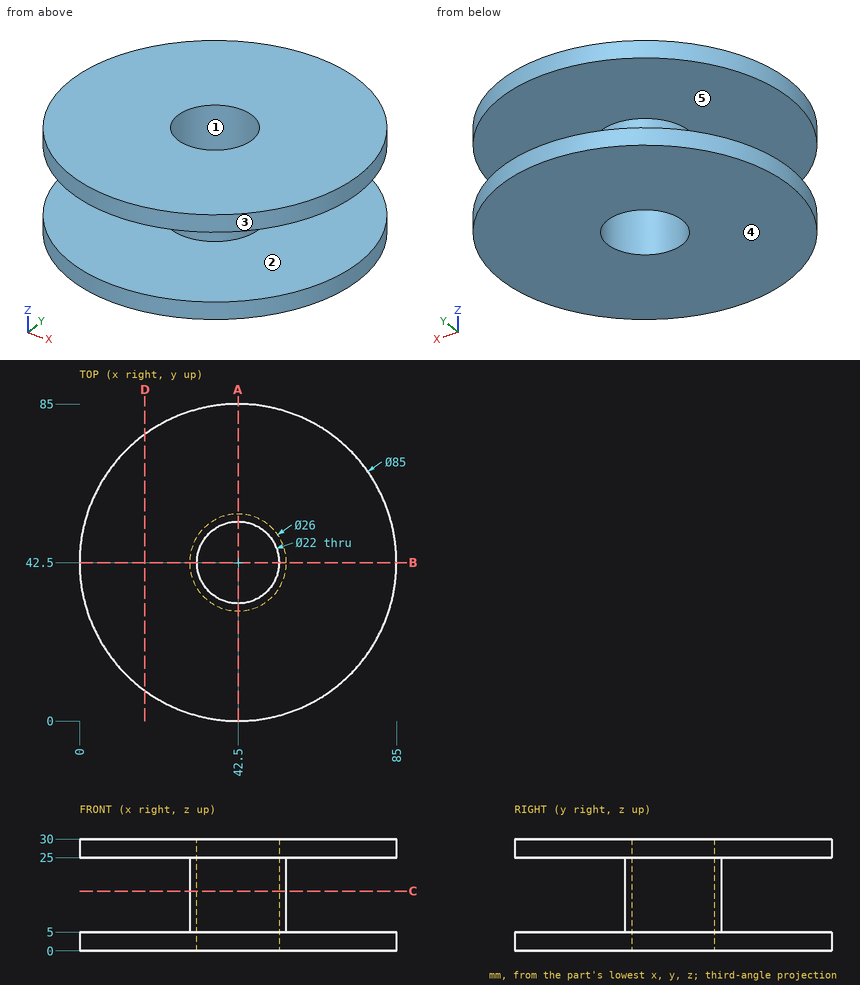
Here's the drawing with two shaded views (mm, measured from the low corner). I have some questions. A direction names the side the tool comes from. Coordinates: 2 decimals unless noted, no trailing zeros. Order: outer loops, then holes, each group sorted by start corner. A loop starts at its lowest first (then second) coordinate and runs counter-clockwise, first axis right, second up.
Item 1: I'm going to push flat-ended pins straight in: pin 1 Ø20 at (x, y) = (42.5, 42.5) entering from -Z; pin 2 Ø1.5 at (y, z) = (38.5, 14.5) entering from -X; pin 3 Ø2 at (x, z) = (45.5, 4) entering from +Y; pin 4 Ø4 at (y, z) = (16.5, 4) entering from -X. Where does each tip first touch, or does it pass through?
Response values:
pin 1: passes through
pin 2: stops at x = 29.91
pin 3: stops at y = 84.95
pin 4: stops at x = 7.43
Item 2: Which directions (+Z, -Z, +X, -X, +Y, -Y) give clear straight access to the entire face, cutting with the end or side of a thin tool? Please do the marked faces 4 and 5.
Response values:
face 4: -Z, +X, -X, +Y, -Y
face 5: none
Item 3: Thinking about a two-plate mould opening in Y: for the marked faces 1, 2 and 3, which applies, pulls with the +Y half, pulls with the -Y half, needs draft (parallel to the pull), parting line crosses it, or undercut?
Response values:
face 1: undercut
face 2: needs draft
face 3: parting line crosses it
Item 4: If we section it at A-A, the plane x = 42.5: List the corners of the cut face in (y, z) for me.
Response values:
outline: (0, 0) - (31.5, 0) - (31.5, 30) - (0, 30) - (0, 25) - (29.5, 25) - (29.5, 5) - (0, 5) - close; (53.5, 0) - (85, 0) - (85, 5) - (55.5, 5) - (55.5, 25) - (85, 25) - (85, 30) - (53.5, 30) - close
Item 5: I need wall thicknesses on probe 1 along Y at (x, z) = (42.5, 9.75); probe 2 along Z at (x, y) = (6.5, 30); probe 3 along Y at (x, z) = (50, 10.75). Which ranges of each line are inside material? Lowest first, please.
Response values:
probe 1: y = 29.5 to 31.5, 53.5 to 55.5
probe 2: z = 0 to 5, 25 to 30
probe 3: y = 31.88 to 34.45, 50.55 to 53.12
Item 6: If we section it at D-D, the plane x = 17.5: List the corners of the cut face in (y, z) for me, then the cut area to 3 significant figures.
Response values:
outline: (8.13, 0) - (76.87, 0) - (76.87, 5) - (8.13, 5) - close; (8.13, 25) - (76.87, 25) - (76.87, 30) - (8.13, 30) - close
area: 687 mm2
Item 7: If we section it at C-C, the plane z = 16: List the corners of the cut face in (x, y) for me, then the cut area to 3 significant figures.
Response values:
outline: circle Ø26 at (42.5, 42.5); hole circle Ø22 at (42.5, 42.5)
area: 151 mm2
